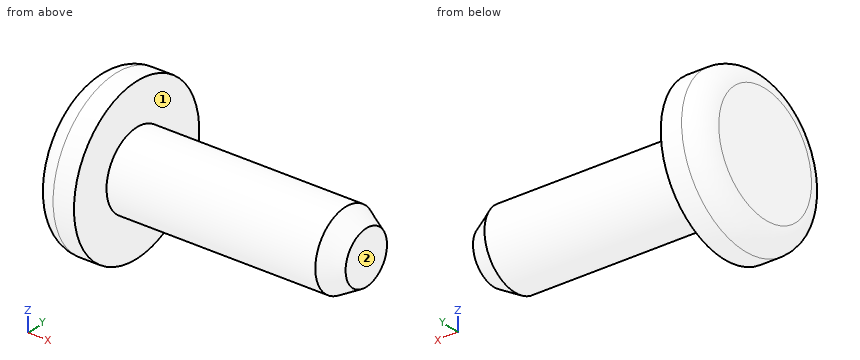
```python
from build123d import *

# Parameters (mm, degrees)
SKETCH1_R           = 2.3495
BOSS_EXTRUDE1_DEPTH = 6.985
CHAMFER1_SIZE       = 1.27
CHAMFER1_SIZE2      = 0.733234842


with BuildPart() as part:
    # Sketch1 → Boss-Extrude1 (new body, symmetric)
    with BuildSketch(Plane(origin=(0, 0, 0), x_dir=(0, 0, -1), z_dir=(1, 0, 0))):
        Circle(SKETCH1_R)
    extrude(amount=BOSS_EXTRUDE1_DEPTH, both=True)

    # Sketch2 → Revolve1 (revolve)
    with BuildSketch(Plane(origin=(0, 0, 0), x_dir=(1, 0, 0), z_dir=(0, 1, 0))):
        with BuildLine():
            Line((-9.525, 0), (-6.985, 0))
            Line((-6.985, 0), (-6.985, -4.8895))
            Line((-6.985, -4.8895), (-8.255, -4.8895))
            ThreePointArc((-8.255, -4.8895), (-9.153025612, -4.517525612), (-9.525, -3.6195))
            Line((-9.525, -3.6195), (-9.525, 0))
        make_face()
    revolve(axis=Axis((-9.525, 0, 0), (1, 0, 0)))

    # Chamfer1
    chamfer1_edges = [part.edges().sort_by_distance(p)[0] for p in [
        (6.985, 0, 2.3495),
    ]]
    chamfer1_side = [part.faces().sort_by_distance(p)[0] for p in [
        (0, 0, 2.3495),
    ]]
    chamfer(chamfer1_edges, length=CHAMFER1_SIZE, length2=CHAMFER1_SIZE2, reference=chamfer1_side[0])


solid = part.part
```
Verification items for the finished model (mm, model axes). Face numbers are marked on the shaded views. A direction names the side the tool comes from. Give positions to 0.01 mm unless a question says otherwise; leave off trailing zeros. Order: outer loops, then holes, each group sorted by start corner. A loop starts at its lowest first (then second) coordinate and runs counter-clockwise, first axis right, second up. Notation, with made-up numbers: M 54.25,84.5 L 107.25,84.5 A22 ccw 107.25,110.5 Z; hole C 74.5,83 d1. An arc over 180 degrees is marked long. Return JSON: item names as keys, results as strings. Group by question number.
1) Section check A-A on z = 0. Record the cut outline in (x, y) (1 decimal).
2) Section check C-C on x = 2.25. Record the cut outline in (y, z).
3) Access from +Z, -Z, +X, -X, +Y, -Y to the whole of each face (thin tool, end or side, straight path). Record for the marked faces 1 and 2.
4) Go/stop test with flat-tipped pins: pin 1 Ø1.5 at (x, y) = (-7, 2.5) entering from +Z; pin 2 Ø4 at (x, z) = (1.5, 3) entering from +Y; pin 3 Ø5 at (x, z) = (0, 1) entering from +Y. Record where each tip stops, or that it passes through.
5) Scan lines: line 1 (X direction, y = -2, z = 3) (3 decimals); line 2 (Y direction, x = 1.75, z = -1); line 3 (X direction, y = -4.5, z = -1) (3 decimals). Record each from-to range of solid material in increasing order.
Answer block:
{
 "1": {"outline": "M -9.5,-3.6 A1.3 ccw -8.3,-4.9 L -7,-4.9 L -7,-2.3 L 5.7,-2.3 L 7,-1.6 L 7,1.6 L 5.7,2.3 L -7,2.3 L -7,4.9 L -8.3,4.9 A1.3 ccw -9.5,3.6 Z"},
 "2": {"outline": "C 0,0 d4.7"},
 "3": {"face 1": "+X", "face 2": "+Z, -Z, +X, +Y, -Y"},
 "4": {"pin 1": "stops at z = 4.57", "pin 2": "stops at y = 2.13", "pin 3": "stops at y = 2.35"},
 "5": {"line 1": "x = -9.525 to -6.985", "line 2": "y = -2.13 to 2.13", "line 3": "x = -9.05 to -6.985"}
}
